```python
from build123d import *

# Parameters (mm, degrees)
SKETCH1_W           = 28.5
SKETCH1_H           = 40
BOSS_EXTRUDE1_DEPTH = 5
SKETCH2_W           = 28.5
SKETCH2_H           = 40
SKETCH2_R           = 2.1
BOSS_EXTRUDE2_DEPTH = 2
CHAMFER1_SIZE       = 6


with BuildPart() as part:
    # Sketch1 → Boss-Extrude1 (new body)
    with BuildSketch(Plane(origin=(0, 0, 444.620141885), x_dir=(-1, 0, 0), z_dir=(0, 0, -1))):
        with Locations((146.960843614, -510.298939869)):
            Rectangle(SKETCH1_W, SKETCH1_H)
        Polygon((149.40344611, -524.327662084), (153.05344611, -522.220333602), (153.05344611, -518.005676636), (149.40344611, -515.898348154), (145.75344611, -518.005676636), (145.75344611, -522.220333602), align=None, mode=Mode.SUBTRACT)
    extrude(amount=BOSS_EXTRUDE1_DEPTH)

    # Sketch2 → Boss-Extrude2 (add)
    with BuildSketch(Plane(origin=(0, 0, 444.620141885), x_dir=(-1, 0, 0), z_dir=(0, 0, -1))):
        with Locations((146.960843614, -510.298939869)):
            Rectangle(SKETCH2_W, SKETCH2_H)
        with Locations((149.40344611, -520.113005119)):
            Circle(SKETCH2_R, mode=Mode.SUBTRACT)
    extrude(amount=BOSS_EXTRUDE2_DEPTH)

    # Chamfer1
    chamfer1_edges = [part.edges().sort_by_distance(p)[0] for p in [
        (-161.210843614, -530.298939869, 442.120141885),
        (-132.710843614, -530.298939869, 442.120141885),
        (-132.710843614, -490.298939869, 442.120141885),
        (-161.210843614, -490.298939869, 442.120141885),
    ]]
    chamfer(chamfer1_edges, length=CHAMFER1_SIZE)


solid = part.part
```
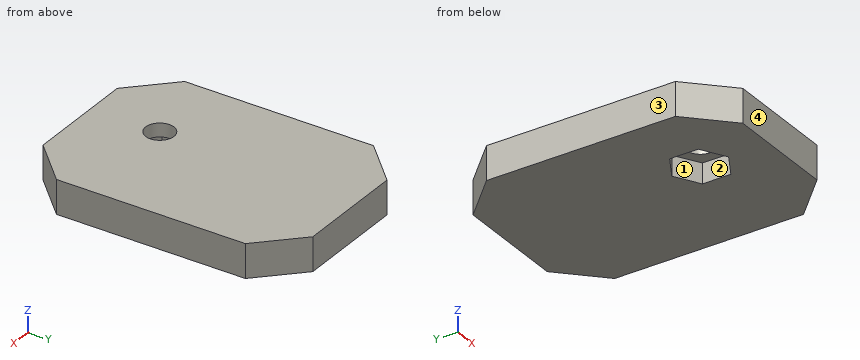
Geometry: final body of the model. Coordinates: model frame, mm. Face numbers are marked on the shaded views. Round coordinates to 2 decimals unless told otherwise and drop trailing zeros. Write each loop counter-clockwise with the first axis right and the second up, starting at its lowest first coordinate (ties: lowest second). Pieces come first, ordered by that corner, then holes.
Item 1: Section query B-B (z = 444.15). Return loops of the section in (x, y).
Item 2: Pin query (flat end, axial travel): P1, Ø4, axis at x = -149.4, y = -520.11, coming from the -Z side; P2, Ø2, axis at x = -150, y = -522, coming from the -Z side. Return the tip coordinate at first contact, or that it passes through.
Item 3: Material intervals for L1, parallel to X at y = -520, z = 442.5; L2, parallel to Y at x = -149.25, z = 443; L3, parallel to Y at x = -148.75, z = 444.35, sorted ascending.
Item 4: Section query A-A (z = 440.4). Return loops of the section in (x, y), plus the area to 3 significant figures.
Item 5: Section query C-C (x = -135.5). Return loops of the section in (y, z).
Item 6: Mould query, pull axis X, two halves, no side actions, for the marked faces 1, 2, 3 and 4. Classes: +X half, -X half, draft (parallel to the pull), parting line (faces both ways), or undercut.
Item 7: Section query D-D (y = -494.5). Return loops of the section in (x, z), plus the area to 3 significant figures.
Completed:
1. outline: (-161.21, -524.3) - (-155.21, -530.3) - (-138.71, -530.3) - (-132.71, -524.3) - (-132.71, -496.3) - (-138.71, -490.3) - (-155.21, -490.3) - (-161.21, -496.3) - close; hole circle Ø4.2 at (-149.4, -520.11)
2. P1: passes through
2. P2: stops at z = 442.62
3. L1: x = -161.21 to -153.05, -145.75 to -132.71
3. L2: y = -530.3 to -522.21, -518.02 to -490.3
3. L3: y = -530.3 to -522.11, -518.12 to -490.3
4. outline: (-161.21, -524.3) - (-155.21, -530.3) - (-138.71, -530.3) - (-132.71, -524.3) - (-132.71, -496.3) - (-138.71, -490.3) - (-155.21, -490.3) - (-161.21, -496.3) - close; hole (-153.05, -522.22) - (-149.4, -524.33) - (-145.75, -522.22) - (-145.75, -518.01) - (-149.4, -515.9) - (-153.05, -518.01) - close
4. area: 1,020 mm2
5. outline: (-527.09, 439.62) - (-493.51, 439.62) - (-493.51, 444.62) - (-527.09, 444.62) - close
6. face 1: undercut
6. face 2: undercut
6. face 3: -X half
6. face 4: draft
7. outline: (-159.41, 439.62) - (-134.51, 439.62) - (-134.51, 444.62) - (-159.41, 444.62) - close
7. area: 125 mm2
